Design review of the part built by this model. Coordinates are the model's own, in mm. A direction names the side the tool comes from. Give positions to 0.01 mm unless a question says otherwise; leave off trailing zeros. Write each loop counter-clockwise with the first axis right and the second up, starting at its lowest first coordinate (ties: lowest second). Pieces come first, ordered by that corner, then holes. Notation, with made-up numbers: M -10.5,86 L 27.5,86 A28 ccw 27.5,115 Z; hole C 82,49 d2. An arc over 180 degrees is marked long. Answer in a Markdown table with one row per item.
```python
from build123d import *

# Parameters (mm, degrees)
SKETCH_4_R          = 6.25
CUT_EXTRUDE_1_DEPTH = 10
SKETCH_5_W          = 4.872533435
SKETCH_5_H          = 19.874807433
CUT_EXTRUDE_2_DEPTH = 8


with BuildPart() as part:
    # 草图3 → 旋转1 (revolve)
    with BuildSketch(Plane.XY):
        Polygon((0, 0), (0, 8), (8, 8), (8, 9), (10, 9), (10, 8), (15.4, 8), (15.4, 0), align=None)
    revolve(axis=Axis((15.4, 0, 0), (-1, 0, 0)))

    # 草图4 → 切除-拉伸1 (cut)
    with BuildSketch(Plane.ZY.offset(-15.4)):
        with Locations(Location((0, 0, 0), (0, 0, 270))):
            Circle(SKETCH_4_R)
    extrude(amount=CUT_EXTRUDE_1_DEPTH, mode=Mode.SUBTRACT)

    # 草图5 → 切除-拉伸2 (cut)
    with BuildSketch(Plane.ZY):
        with Locations((9.686266718, -0.512898256)):
            Rectangle(SKETCH_5_W, SKETCH_5_H)
        with Locations((-9.686266718, -0.512898256)):
            Rectangle(SKETCH_5_W, SKETCH_5_H)
    extrude(amount=-CUT_EXTRUDE_2_DEPTH, mode=Mode.SUBTRACT)


solid = part.part
```
1) To check wall thickness, follow probe 1 along Z at (x, y) = (10.75, 0); probe 2 along Z at (x, y) = (9.25, 0); probe 3 along X at (y, z) = (1.25, 7.5). State the ranges of each line that lie inside material, in increasing order. Write a range as [from, to].
Geometry says:
| item | result |
|---|---|
| probe 1 | [-8, -6.25], [6.25, 8] |
| probe 2 | [-9, -6.25], [6.25, 9] |
| probe 3 | [8, 15.4] |
2) Add section B-B (x = 9). Write out the cut boundary in (y, z).
Geometry says:
| item | result |
|---|---|
| outline | C 0,0 d18; hole C 0,0 d12.5 |
3) Insertion check: P1, Ø6, axis at y = 0.5, z = -2, coming from the +X side; P2, Ø1, axis at x = 4, y = 4.5, coming from the -Z side; P3, Ø2, axis at x = 3, y = 0, coming from the +Z side. Each pin has a flat end and moves straight along its axis. Give the tip position at first contact, or say it passes through.
Geometry says:
| item | result |
|---|---|
| P1 | x = 5.4 |
| P2 | z = -6.93 |
| P3 | z = 7.25 |
4) The part is to be moulded in two halves that separate along Y. For faces 5 (the face through (4, -8, 0)), 6 (the face through (4, 0, -7.25)), 7 (the face through (5.4, 0, 0)), say which applies: released by +Y, released by -Y, zero draft, split by the parting line, or undercut.
Geometry says:
| item | result |
|---|---|
| face 5 | released by -Y |
| face 6 | zero draft |
| face 7 | undercut |
5) For faces 1 (the face through (4, 0, 7.25)), 2 (the face through (4, 8, 0)), 3 (the face through (12.74, -1.73, 7.81)), 4 (the face through (0, 0, 0)), list the 3-axis set-ups (+Z, -Z, +X, -X, +Y, -Y) from which the entire face can be reached by the end or side of a thin tool; tool diameter is ignored.
Geometry says:
| item | result |
|---|---|
| face 1 | +Z, -X, +Y, -Y |
| face 2 | -X, +Y |
| face 3 | +X |
| face 4 | +Z, -Z, -X, +Y, -Y |
6) Add section A-A (z = 0). Write out the cut boundary in (x, y).
Geometry says:
| item | result |
|---|---|
| outline | M 0,-8 L 8,-8 L 8,-9 L 10,-9 L 10,-8 L 15.4,-8 L 15.4,-6.25 L 5.4,-6.25 L 5.4,6.25 L 15.4,6.25 L 15.4,8 L 10,8 L 10,9 L 8,9 L 8,8 L 0,8 Z |
7) Add section D-D (x = 2.5). Write out the cut boundary in (y, z).
Geometry says:
| item | result |
|---|---|
| outline | M -3.38,-7.25 L 3.38,-7.25 A8 ccw 3.38,7.25 L -3.38,7.25 A8 ccw Z |
8) Add section C-C (y = 0). Write out the cut boundary in (x, z).
Geometry says:
| item | result |
|---|---|
| outline | M 0,-7.25 L 8,-7.25 L 8,-9 L 10,-9 L 10,-8 L 15.4,-8 L 15.4,-6.25 L 5.4,-6.25 L 5.4,6.25 L 15.4,6.25 L 15.4,8 L 10,8 L 10,9 L 8,9 L 8,7.25 L 0,7.25 Z |
